Input: part model. Units: mm. Frame: model coordinates. A direction names the side the tool comes from. Give positions to 0.01 mm unless a question says otherwise; leave off trailing zeros. Loops run counter-clockwise (first coordinate to the right, second up) from the corner with the lowest first, then second, coordinate; pieces in that order, holes last. Notation, with made-up numbers: M 49,4.25 L 56,4.25 A22 ccw 56,13.25 Z; hole C 29,39.5 d2. An arc over 180 degrees is marked long. Use CSV: the item, a comma, the result in double quotes. Start each with the question number.
Q1. Section C-C, the plane y = 1.45. Output: boundary loops of the cut face in (x, z), plus the area to 3 significant figures.
Q2. Pull-direction query (X, two-part tool) for faces 4 (the flat face through (7, 1, -5)), 5 (the flat face through (-3, 1, -8)), 6 (the cylindrical face through (-0.6, 1.5, -4.3)), 7 (the flat face through (5, 1, -7)); classes: released by +X, released by -X, zero draft, split by the parting line, or undercut.
Q3. Section A-A, the plane z = -3.5. Output: boundary loops of the cut face in (x, y), plus the area to 3 significant figures.
Q4. Section D-D, the plane z = -7.75. Output: boundary loops of the cut face in (x, y), plus the area to 3 significant figures.
Q5. Reachability of faces 1 (the flat face through (3, 1, -9)), 2 (the flat face through (-5, 1, -7)), 3 (the flat face through (0, 0, -5)) from +Z, -Z, +X, -X, +Y, -Y: full face, straight path, thin tool, end or side. Return the list, or none.
Q6. Pin query (flat end, axial travel): pin 1 (1.5 mm diameter, centred on x = -5.5, y = 1, fed in from -Z); pin 2 (1.5 mm diameter, centred on y = 1.5, z = -8.5, fed in from -X). Return the tip coordinate at first contact, or that it passes through.
Q7. Material intervals for line 1 along X through (y, z) = (1.75, -3.5); line 2 along X through (y, z) = (2.4, -8.25); line 3 along X through (y, z) = (1, -4.25), sorted ascending.
Q8. Section B-B, the plane x = 0. Output: boundary loops of the cut face in (y, z).
from build123d import *

# Parameters (mm, degrees)
ESQUISSE1_R        = 1
BOSS_EXTRU_1_DEPTH = 3


with BuildPart() as part:
    # Esquisse1 → Boss.-Extru.1 (new body)
    with BuildSketch(Plane(origin=(0, 0, 0), x_dir=(1, 0, 0), z_dir=(0, 1, 0))):
        with BuildLine():
            Line((-7, 7), (-3, 7))
            Line((-3, 7), (-3, 10))
            Line((-3, 10), (3, 10))
            Line((3, 10), (3, 7))
            Line((3, 7), (7, 7))
            Line((7, 7), (7, 3))
            ThreePointArc((7, 3), (6.121320344, 0.878679656), (4, 0))
            Line((4, 0), (-4, 0))
            ThreePointArc((-4, 0), (-6.121320344, 0.878679656), (-7, 3))
            Line((-7, 3), (-7, 7))
        make_face()
        with Locations(Location((0, 3.5, 0), (0, 0, 270))):
            Circle(ESQUISSE1_R, mode=Mode.SUBTRACT)
    extrude(amount=BOSS_EXTRU_1_DEPTH)


solid = part.part
A:
1,outline,"M -7,-7 L -3,-7 L -3,-10 L 3,-10 L 3,-7 L 7,-7 L 7,-3 A3 ccw 4,0 L -4,0 A3 ccw -7,-3 Z; hole C 0,-3.5 d2"
1,area,"109 mm^2"
2,face 4,"released by +X"
2,face 5,"released by -X"
2,face 6,"undercut"
2,face 7,"zero draft"
3,outline,"M -7,0 L -1,0 L -1,3 L -7,3 Z; M 1,0 L 7,0 L 7,3 L 1,3 Z"
3,area,"36.0 mm^2"
4,outline,"M -3,0 L 3,0 L 3,3 L -3,3 Z"
4,area,"18.0 mm^2"
5,face 1,"-Z, +X, +Y, -Y"
5,face 2,"-Z, -X, +Y, -Y"
5,face 3,"+Z, -Z, +X, -X, -Y"
6,pin 1,"z = -7"
6,pin 2,"x = -3"
7,line 1,"-7 to -1, 1 to 7"
7,line 2,"-3 to 3"
7,line 3,"-7 to -0.66, 0.66 to 7"
8,outline,"M 0,-10 L 3,-10 L 3,-4.5 L 0,-4.5 Z; M 0,-2.5 L 3,-2.5 L 3,0 L 0,0 Z"
